from build123d import *

# Parameters (mm, degrees)
SKETCH2_R           = 20
SKETCH2_R_2         = 2.325
BOSS_EXTRUDE1_DEPTH = 3
SKETCH3_W           = 3
SKETCH3_H           = 1.5


with BuildPart() as part:
    # Sketch2 → Boss-Extrude1 (new body)
    with BuildSketch(Plane(origin=(0, 0, 0), x_dir=(1, 0, 0), z_dir=(0, 1, 0))):
        with Locations(Location((0, 0, 0), (0, 0, 270))):
            Circle(SKETCH2_R)
        with Locations(Location((0, 0, 0), (0, 0, 270))):
            Circle(SKETCH2_R_2, mode=Mode.SUBTRACT)
        with BuildLine():
            Line((-1.302361333, 7.386058148), (-2.604722665, 14.772116295))
            ThreePointArc((-2.604722665, 14.772116295), (-8.816778784, 12.135254916), (-13.244213893, 7.042073442))
            Line((-13.244213893, 7.042073442), (-6.622106946, 3.521036721))
            ThreePointArc((-6.622106946, 3.521036721), (-4.408389392, 6.067627458), (-1.302361333, 7.386058148))
        make_face(mode=Mode.SUBTRACT)
        with BuildLine():
            Line((1.302361333, 7.386058148), (2.604722665, 14.772116295))
            ThreePointArc((2.604722665, 14.772116295), (8.816778784, 12.135254916), (13.244213893, 7.042073442))
            Line((13.244213893, 7.042073442), (6.622106946, 3.521036721))
            ThreePointArc((6.622106946, 3.521036721), (4.408389392, 6.067627458), (1.302361333, 7.386058148))
        make_face(mode=Mode.SUBTRACT)
        with BuildLine():
            Line((7.427010516, 1.043798257), (14.854021031, 2.087596514))
            ThreePointArc((14.854021031, 2.087596514), (14.265847744, -4.635254916), (10.790097005, -10.419875557))
            Line((10.790097005, -10.419875557), (5.395048503, -5.209937778))
            ThreePointArc((5.395048503, -5.209937778), (7.132923872, -2.317627458), (7.427010516, 1.043798257))
        make_face(mode=Mode.SUBTRACT)
        with BuildLine():
            Line((3.287783601, -6.740955347), (6.575567202, -13.481910694))
            ThreePointArc((6.575567202, -13.481910694), (0, -15), (-6.575567202, -13.481910694))
            Line((-6.575567202, -13.481910694), (-3.287783601, -6.740955347))
            ThreePointArc((-3.287783601, -6.740955347), (0, -7.5), (3.287783601, -6.740955347))
        make_face(mode=Mode.SUBTRACT)
        with BuildLine():
            Line((-5.395048503, -5.209937778), (-10.790097005, -10.419875557))
            ThreePointArc((-10.790097005, -10.419875557), (-14.265847744, -4.635254916), (-14.854021031, 2.087596514))
            Line((-14.854021031, 2.087596514), (-7.427010516, 1.043798257))
            ThreePointArc((-7.427010516, 1.043798257), (-7.132923872, -2.317627458), (-5.395048503, -5.209937778))
        make_face(mode=Mode.SUBTRACT)
    extrude(amount=BOSS_EXTRUDE1_DEPTH)

    # Sketch3 → Cut-Revolve1 (revolve, cut)
    with BuildSketch(Plane.XY, mode=Mode.PRIVATE) as cut_revolve1_sk:
        with Locations((18.5, 1.5)):
            Rectangle(SKETCH3_W, SKETCH3_H)
    revolve(cut_revolve1_sk.sketch.rotate(Axis((0, 0, 0), (0, 1, 0)), 90), axis=Axis((0, 0, 0), (0, 1, 0)), mode=Mode.SUBTRACT)


solid = part.part
Could you check a few things on this model? Use its own coordinates, in mm. Give positions to 0.01 mm unless a question says otherwise; leave off trailing zeros. Order: outer loops, then holes, each group sorted by start corner. A loop starts at its lowest first (then second) coordinate and runs counter-clockwise, first axis right, second up. Notation, with made-up numbers: (5.5, 36) -> (61.5, 36) arc R18 cw to (61.5, 59) -> close; hole circle Ø6 at (65, -37). An arc over 180 degrees is marked (long way). Answer in a Markdown table with one row per item. Add a question column.
Item 1: We'd pull the mould along Y, two halves only. Please class faces 1 (the flat face through (15, 0.75, -9)), 2 (the cylindrical face through (9, 1, -12)), 3 (the flat face through (-4, 0, 0)), 4 (the flat face through (-4, 3, 0)): pulls with the +Y half, pulls with the -Y half, needs draft (parallel to the pull), parting line crosses it, or undercut.
Item 2: Imagine slicing it at B-B (y = 1.2). List the corners of the cut face in (x, z) for me (3 decimals), and give its area (3 significant figures).
Item 3: Imagine slicing it at C-C (z = 0). List the corners of the cut face in (x, y) for me (3 decimals), and give its area (4 significant figures).
Item 4: Imagine slicing it at D-D (z = 14.5). List the corners of the cut face in (x, y) for me, and give its area (3 significant figures).
Item 5: I'm going to push flat-ended pins straight in: P1, Ø12, axis at x = 12.5, z = 8, coming from the -Y side; P2, Ø3.5, axis at x = 0, z = 0, coming from the +Y side; P3, Ø1.5, axis at x = -12.5, y = 2, coming from the -Z side. Where does each tip first touch, or does it pass through?
Item 6: Please list where these lines run through material, in increasing order: probe 1 along X at (y, z) = (0.9, 0) (3 decimals); probe 2 along Y at (x, z) = (3, -17.5); probe 3 along X at (y, z) = (0.95, -13.5).
Item 7: Imagine slicing it at A-A (x = 0). List the corners of the cut face in (y, z) for me (3 decimals), and give its area (4 significant figures).
Result:
| question | item | result |
|---|---|---|
| 1 | face 1 | undercut |
| 1 | face 2 | needs draft |
| 1 | face 3 | pulls with the -Y half |
| 1 | face 4 | pulls with the +Y half |
| 2 | outline | circle Ø34 at (0, 0); hole (-14.854, -2.088) -> (-7.427, -1.044) arc R7.5 cw to (-5.395, 5.21) -> (-10.79, 10.42) arc R15 ccw to start; hole (-13.244, -7.042) arc R15 ccw to (-2.605, -14.772) -> (-1.302, -7.386) arc R7.5 cw to (-6.622, -3.521) -> close; hole (-6.576, 13.482) -> (-3.288, 6.741) arc R7.5 cw to (3.288, 6.741) -> (6.576, 13.482) arc R15 ccw to start; hole circle Ø4.65 at (0, 0); hole (1.302, -7.386) -> (2.605, -14.772) arc R15 ccw to (13.244, -7.042) -> (6.622, -3.521) arc R7.5 cw to start; hole (5.395, 5.21) arc R7.5 cw to (7.427, -1.044) -> (14.854, -2.088) arc R15 ccw to (10.79, 10.42) -> close |
| 2 | area | 508 mm2 |
| 3 | outline | (-20, 0) -> (-15, 0) -> (-15, 3) -> (-20, 3) -> (-20, 2.25) -> (-17, 2.25) -> (-17, 0.75) -> (-20, 0.75) -> close; (-7.5, 0) -> (-2.325, 0) -> (-2.325, 3) -> (-7.5, 3) -> close; (2.325, 0) -> (7.5, 0) -> (7.5, 3) -> (2.325, 3) -> close; (15, 0) -> (20, 0) -> (20, 0.75) -> (17, 0.75) -> (17, 2.25) -> (20, 2.25) -> (20, 3) -> (15, 3) -> close |
| 3 | area | 52.05 mm2 |
| 4 | outline | (-13.77, 0) -> (-3.84, 0) -> (-3.84, 3) -> (-13.77, 3) -> (-13.77, 2.25) -> (-8.87, 2.25) -> (-8.87, 0.75) -> (-13.77, 0.75) -> close; (3.84, 0) -> (13.77, 0) -> (13.77, 0.75) -> (8.87, 0.75) -> (8.87, 2.25) -> (13.77, 2.25) -> (13.77, 3) -> (3.84, 3) -> close |
| 4 | area | 44.9 mm2 |
| 5 | P1 | y = 0 |
| 5 | P2 | through |
| 5 | P3 | z = -16.15 |
| 6 | probe 1 | -17 to -15, -7.5 to -2.325, 2.325 to 7.5, 15 to 17 |
| 6 | probe 2 | 0 to 0.75, 2.25 to 3 |
| 6 | probe 3 | -10.33 to -6.54, -2.38 to 2.38, 6.54 to 10.33 |
| 7 | outline | (0, -20) -> (0.75, -20) -> (0.75, -17) -> (2.25, -17) -> (2.25, -20) -> (3, -20) -> (3, -2.325) -> (0, -2.325) -> close; (0, 2.325) -> (3, 2.325) -> (3, 7.5) -> (0, 7.5) -> close; (0, 15) -> (3, 15) -> (3, 20) -> (2.25, 20) -> (2.25, 17) -> (0.75, 17) -> (0.75, 20) -> (0, 20) -> close |
| 7 | area | 74.55 mm2 |
